```python
from build123d import *

# Parameters (mm, degrees)
SKETCH1_R           = 14.2875
SKETCH1_R_2         = 3.175
BOSS_EXTRUDE1_DEPTH = 3.175
FILLET1_R           = 3.81


with BuildPart() as part:
    # Sketch1 → Boss-Extrude1 (new body)
    with BuildSketch(Plane.XY):
        Polygon((0, 0), (0, 127), (25.4, 127), (101.6, 76.2), (101.6, 0), align=None)
        with Locations((57.15, 76.2)):
            Circle(SKETCH1_R, mode=Mode.SUBTRACT)
        with Locations((12.7, 12.7)):
            Circle(SKETCH1_R_2, mode=Mode.SUBTRACT)
        with Locations((38.1, 12.7)):
            Circle(SKETCH1_R_2, mode=Mode.SUBTRACT)
        with Locations((63.5, 12.7)):
            Circle(SKETCH1_R_2, mode=Mode.SUBTRACT)
        with Locations((88.9, 12.7)):
            Circle(SKETCH1_R_2, mode=Mode.SUBTRACT)
        with Locations((12.7, 38.1)):
            Circle(SKETCH1_R_2, mode=Mode.SUBTRACT)
        with Locations((12.7, 63.5)):
            Circle(SKETCH1_R_2, mode=Mode.SUBTRACT)
        with Locations((12.7, 88.9)):
            Circle(SKETCH1_R_2, mode=Mode.SUBTRACT)
        with Locations((12.7, 114.3)):
            Circle(SKETCH1_R_2, mode=Mode.SUBTRACT)
    extrude(amount=BOSS_EXTRUDE1_DEPTH)

    # Fillet1
    fillet1_edges = [part.edges().sort_by_distance(p)[0] for p in [
        (0, 0, 1.5875),
        (0, 127, 1.5875),
        (25.4, 127, 1.5875),
        (101.6, 76.2, 1.5875),
        (101.6, 0, 1.5875),
    ]]
    fillet(fillet1_edges, radius=FILLET1_R)


solid = part.part
```
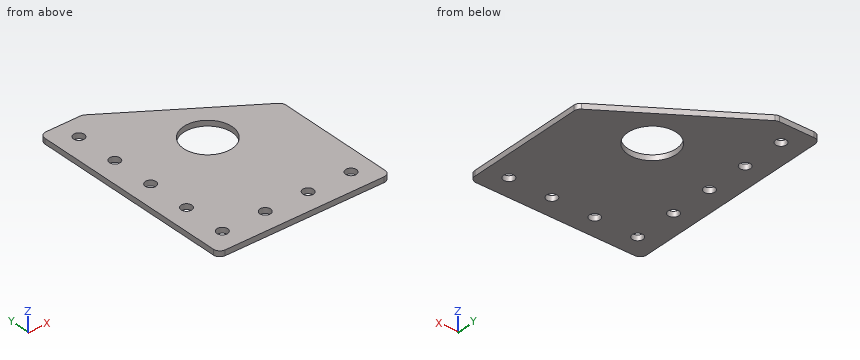
Geometry check sheet. Reference: the model listing, model coordinates, mm. Coordinates: 2 decimals unless noted, no trailing zeros. Order: outer loops, then holes, each group sorted by start corner. A loop starts at its lowest first (then second) coordinate and runs counter-clockwise, first axis right, second up.
Item 1: Scan lines: line 1 along Y through (x, z) = (12.7, 2.1) (3 decimals); line 2 along Y through (x, z) = (10.5, 3); line 3 along X through (y, z) = (75, 2.1). Record each from-to range of solid material in increasing order.
Item 2: Section check A-A (y = 114.3). Enter the section's corners in (x, z) (3 decimals), plus the area to 3 significant figures.
Item 3: Depth check by flat-ended pin: pin 1 (10 mm diameter, centred on x = 12.7, y = 12.7, fed in from -Z); pin 2 (5 mm diameter, centred on x = 12.7, y = 88.9, fed in from +Z); pin 3 (1.5 mm diameter, centred on x = 37.5, z = 1.5, fed in from +Y). Enter the tip coordinate at first touch or a pass-through.
Item 4: Section check B-B (z = 2.3). Count the separate pieces of the cut face and the enclosed holes in it, plus the area to 3 significant figures.
Item 5: Section check D-D (y = 63.5). Enter the section's corners in (x, z) (3 decimals), plus the area to 3 significant figures.
Item 6: Section check C-C (x = 36.5). Enter the section's corners in (y, z) (3 decimals).
Check sheet entries:
1. line 1: y = 0 to 9.525, 15.875 to 34.925, 41.275 to 60.325, 66.675 to 85.725, 92.075 to 111.125, 117.475 to 127
1. line 2: y = 0 to 10.41, 14.99 to 35.81, 40.39 to 61.21, 65.79 to 86.61, 91.19 to 112.01, 116.59 to 127
1. line 3: x = 0 to 42.91, 71.39 to 101.51
2. outline: (0, 0) - (9.525, 0) - (9.525, 3.175) - (0, 3.175) - close; (15.875, 0) - (44.45, 0) - (44.45, 3.175) - (15.875, 3.175) - close
2. area: 121 mm2
3. pin 1: stops at z = 0
3. pin 2: passes through
3. pin 3: stops at y = 119.43
4. separate pieces: 1
4. enclosed holes: 9
4. area: 10,100 mm2
5. outline: (0, 0) - (9.525, 0) - (9.525, 3.175) - (0, 3.175) - close; (15.875, 0) - (50.605, 0) - (50.605, 3.175) - (15.875, 3.175) - close; (63.695, 0) - (101.6, 0) - (101.6, 3.175) - (63.695, 3.175) - close
5. area: 261 mm2
6. outline: (0, 0) - (9.958, 0) - (9.958, 3.175) - (0, 3.175) - close; (15.442, 0) - (119.6, 0) - (119.6, 3.175) - (15.442, 3.175) - close
